```python
from build123d import *

# Parameters (mm, degrees)
SKETCH1_W           = 70
SKETCH1_H           = 154.713144252
SKETCH1_R           = 2.75
SKETCH1_R_2         = 14
BOSS_EXTRUDE1_DEPTH = 5
SKETCH1_4_W         = 70
SKETCH1_4_H         = 154.713144252
SKETCH1_4_R         = 2.75
SKETCH1_4_R_2       = 14
SKETCH1_4_H_2       = 118
SKETCH1_4_R_3       = 5
BOSS_EXTRUDE2_DEPTH = 5
SKETCH2_W           = 70
SKETCH2_H           = 57.356572126
CUT_EXTRUDE1_DEPTH  = 10


with BuildPart() as part:
    # Sketch1 → Boss-Extrude1 (new body)
    with BuildSketch(Plane.XY):
        with Locations((-1.450472168, 0)):
            Rectangle(SKETCH1_W, SKETCH1_H)
        with Locations((-18.5, 57.356572126)):
            Circle(SKETCH1_R, mode=Mode.SUBTRACT)
        with Locations((18.5, 57.356572126)):
            Circle(SKETCH1_R, mode=Mode.SUBTRACT)
        with Locations((-26.450472168, 10)):
            Circle(SKETCH1_R, mode=Mode.SUBTRACT)
        with Locations((26.450472168, 10)):
            Circle(SKETCH1_R, mode=Mode.SUBTRACT)
        with Locations((26.450472168, -10)):
            Circle(SKETCH1_R, mode=Mode.SUBTRACT)
        with Locations((-26.450472168, -10)):
            Circle(SKETCH1_R, mode=Mode.SUBTRACT)
        with Locations((0, 57.356572126)):
            Circle(SKETCH1_R_2, mode=Mode.SUBTRACT)
        with BuildLine():
            Line((-13.95, -33.643427874), (-13.95, -40.643427874))
            ThreePointArc((-13.95, -40.643427874), (-15.5, -42.193427874), (-17.05, -40.643427874))
            Line((-17.05, -40.643427874), (-17.05, -33.643427874))
            ThreePointArc((-17.05, -33.643427874), (-15.5, -32.093427874), (-13.95, -33.643427874))
        make_face(mode=Mode.SUBTRACT)
        with BuildLine():
            Line((17.05, -33.643427874), (17.05, -40.643427874))
            ThreePointArc((17.05, -40.643427874), (15.5, -42.193427874), (13.95, -40.643427874))
            Line((13.95, -40.643427874), (13.95, -33.643427874))
            ThreePointArc((13.95, -33.643427874), (15.5, -32.093427874), (17.05, -33.643427874))
        make_face(mode=Mode.SUBTRACT)
        with BuildLine():
            Line((17.05, -64.643427874), (17.05, -71.643427874))
            ThreePointArc((17.05, -71.643427874), (15.5, -73.193427874), (13.95, -71.643427874))
            Line((13.95, -71.643427874), (13.95, -64.643427874))
            ThreePointArc((13.95, -64.643427874), (15.5, -63.093427874), (17.05, -64.643427874))
        make_face(mode=Mode.SUBTRACT)
        with BuildLine():
            Line((-13.95, -64.643427874), (-13.95, -71.643427874))
            ThreePointArc((-13.95, -71.643427874), (-15.5, -73.193427874), (-17.05, -71.643427874))
            Line((-17.05, -71.643427874), (-17.05, -64.643427874))
            ThreePointArc((-17.05, -64.643427874), (-15.5, -63.093427874), (-13.95, -64.643427874))
        make_face(mode=Mode.SUBTRACT)
        with BuildLine():
            Line((-12, -56.143427874), (-12, -49.143427874))
            ThreePointArc((-12, -49.143427874), (0, -37.143427874), (12, -49.143427874))
            Line((12, -49.143427874), (12, -56.143427874))
            ThreePointArc((12, -56.143427874), (0, -68.143427874), (-12, -56.143427874))
        make_face(mode=Mode.SUBTRACT)
    extrude(amount=BOSS_EXTRUDE1_DEPTH)

    # Sketch1_4 → Boss-Extrude2 (add)
    # profile 1 of 3: a face of its own
    with BuildSketch(Plane.XY):
        with Locations((-1.450472168, 0)):
            Rectangle(SKETCH1_4_W, SKETCH1_4_H)
        with Locations((-26.450472168, -10)):
            Circle(SKETCH1_4_R, mode=Mode.SUBTRACT)
        with BuildLine():
            ThreePointArc((-17.05, -64.643427874), (-15.5, -63.093427874), (-13.95, -64.643427874))
            Line((-13.95, -64.643427874), (-13.95, -71.643427874))
            ThreePointArc((-13.95, -71.643427874), (-15.5, -73.193427874), (-17.05, -71.643427874))
            Line((-17.05, -71.643427874), (-17.05, -64.643427874))
        make_face(mode=Mode.SUBTRACT)
        with BuildLine():
            ThreePointArc((-17.05, -33.643427874), (-15.5, -32.093427874), (-13.95, -33.643427874))
            Line((-13.95, -33.643427874), (-13.95, -40.643427874))
            ThreePointArc((-13.95, -40.643427874), (-15.5, -42.193427874), (-17.05, -40.643427874))
            Line((-17.05, -40.643427874), (-17.05, -33.643427874))
        make_face(mode=Mode.SUBTRACT)
        with Locations((-26.450472168, 10)):
            Circle(SKETCH1_4_R, mode=Mode.SUBTRACT)
        with Locations((-18.5, 57.356572126)):
            Circle(SKETCH1_4_R, mode=Mode.SUBTRACT)
        with BuildLine():
            ThreePointArc((12, -56.143427874), (0, -68.143427874), (-12, -56.143427874))
            Line((-12, -56.143427874), (-12, -49.143427874))
            ThreePointArc((-12, -49.143427874), (0, -37.143427874), (12, -49.143427874))
            Line((12, -49.143427874), (12, -56.143427874))
        make_face(mode=Mode.SUBTRACT)
        with BuildLine():
            ThreePointArc((13.95, -64.643427874), (15.5, -63.093427874), (17.05, -64.643427874))
            Line((17.05, -64.643427874), (17.05, -71.643427874))
            ThreePointArc((17.05, -71.643427874), (15.5, -73.193427874), (13.95, -71.643427874))
            Line((13.95, -71.643427874), (13.95, -64.643427874))
        make_face(mode=Mode.SUBTRACT)
        with BuildLine():
            ThreePointArc((13.95, -33.643427874), (15.5, -32.093427874), (17.05, -33.643427874))
            Line((17.05, -33.643427874), (17.05, -40.643427874))
            ThreePointArc((17.05, -40.643427874), (15.5, -42.193427874), (13.95, -40.643427874))
            Line((13.95, -40.643427874), (13.95, -33.643427874))
        make_face(mode=Mode.SUBTRACT)
        with Locations((26.450472168, -10)):
            Circle(SKETCH1_4_R, mode=Mode.SUBTRACT)
        with Locations((0, 57.356572126)):
            Circle(SKETCH1_4_R_2, mode=Mode.SUBTRACT)
        with Locations((26.450472168, 10)):
            Circle(SKETCH1_4_R, mode=Mode.SUBTRACT)
        with Locations((18.5, 57.356572126)):
            Circle(SKETCH1_4_R, mode=Mode.SUBTRACT)
    # profile 2 of 3: a face of its own
    with BuildSketch(Plane.XY):
        with Locations((-1.450472168, 136.356572126)):
            Rectangle(SKETCH1_4_W, SKETCH1_4_H_2)
        with Locations((-16.991825546, 182.387739686)):
            Circle(SKETCH1_4_R, mode=Mode.SUBTRACT)
        with BuildLine():
            ThreePointArc((-6, 119.856572126), (0, 125.856572126), (6, 119.856572126))
            Line((6, 119.856572126), (6, 94.856572126))
            ThreePointArc((6, 94.856572126), (0, 88.856572126), (-6, 94.856572126))
            Line((-6, 94.856572126), (-6, 119.856572126))
        make_face(mode=Mode.SUBTRACT)
        with Locations((14.09088121, 182.387739686)):
            Circle(SKETCH1_4_R, mode=Mode.SUBTRACT)
    # profile 3 of 3: a face of its own
    with BuildSketch(Plane.XY):
        with Locations((0, 57.356572126)):
            Circle(SKETCH1_4_R_3)
    extrude(amount=BOSS_EXTRUDE2_DEPTH)


with BuildPart() as boss_extrude2_kept_piece:
    # of the separate pieces the step leaves, the one the design keeps (boss_extrude2_pieces_kept)
    add(part.part.solids().sort_by_distance((-36.450472168, -77.356572126, 0))[0])

    # Sketch2 → Cut-Extrude1 (cut)
    with BuildSketch(Plane.XY.offset(5)):
        with Locations((-1.450472168, -48.678286063)):
            Rectangle(SKETCH2_W, SKETCH2_H)
        with BuildLine():
            Line((-13.95, -64.643427874), (-13.95, -71.643427874))
            ThreePointArc((-13.95, -71.643427874), (-15.5, -73.193427874), (-17.05, -71.643427874))
            Line((-17.05, -71.643427874), (-17.05, -64.643427874))
            ThreePointArc((-17.05, -64.643427874), (-15.5, -63.093427874), (-13.95, -64.643427874))
        make_face(mode=Mode.SUBTRACT)
        with BuildLine():
            Line((-13.95, -33.643427874), (-13.95, -40.643427874))
            ThreePointArc((-13.95, -40.643427874), (-15.5, -42.193427874), (-17.05, -40.643427874))
            Line((-17.05, -40.643427874), (-17.05, -33.643427874))
            ThreePointArc((-17.05, -33.643427874), (-15.5, -32.093427874), (-13.95, -33.643427874))
        make_face(mode=Mode.SUBTRACT)
        with BuildLine():
            Line((-12, -56.143427874), (-12, -49.143427874))
            ThreePointArc((-12, -49.143427874), (0, -37.143427874), (12, -49.143427874))
            Line((12, -49.143427874), (12, -56.143427874))
            ThreePointArc((12, -56.143427874), (0, -68.143427874), (-12, -56.143427874))
        make_face(mode=Mode.SUBTRACT)
        with BuildLine():
            Line((17.05, -64.643427874), (17.05, -71.643427874))
            ThreePointArc((17.05, -71.643427874), (15.5, -73.193427874), (13.95, -71.643427874))
            Line((13.95, -71.643427874), (13.95, -64.643427874))
            ThreePointArc((13.95, -64.643427874), (15.5, -63.093427874), (17.05, -64.643427874))
        make_face(mode=Mode.SUBTRACT)
        with BuildLine():
            Line((17.05, -33.643427874), (17.05, -40.643427874))
            ThreePointArc((17.05, -40.643427874), (15.5, -42.193427874), (13.95, -40.643427874))
            Line((13.95, -40.643427874), (13.95, -33.643427874))
            ThreePointArc((13.95, -33.643427874), (15.5, -32.093427874), (17.05, -33.643427874))
        make_face(mode=Mode.SUBTRACT)
    extrude(amount=-CUT_EXTRUDE1_DEPTH, mode=Mode.SUBTRACT)


solid = boss_extrude2_kept_piece.part
```
Input: part model. Units: mm. Frame: model coordinates. A direction names the side the tool comes from. Coordinates: 2 decimals unless noted, no trailing zeros. Loops run counter-clockwise (first coordinate to the right, second up) from the corner with the lowest first, then second, coordinate; pieces in that order, holes last. Notation, with made-up numbers: M 10,31.5 L 40,31.5 A4 ccw 40,36.5 Z; hole C 87,30 d10. An arc over 180 degrees is marked long. Use a Markdown table: item, result. Add a question column.
1) Section B-B, the plane x = 0. Return the cut outline in (y, z).
2) Section C-C, the plane x = -11. Return the cut outline in (y, z).
3) Section A-A, the plane y = 10. Return the cut outline in (x, z), plus the area to 3 significant figures.
4) Line query: L1, parallel to Y at x = -26.5, z = 4.4; L2, parallel to X at y = 8, z = 3.4; L3, parallel to Y at x = -18.5, z = 2.3. Output: solid intervals per line, ascending. Write a range as from..to.
5) Section D-D, the plane z = 3.6. Give the number of separate pieces and of enclosed holes in the cut face, plus the area to 3 significant figures.
6) Draft query along Y for faces 3 (the flat face through (-2, 195.357, 2)), 4 (the cylindrical face through (-20.68, 55.68, 2.46)), 5 (the flat face through (33.55, 86, 2)), 6 (the flat face through (6, 108, 2)). Return one class per face: +Y half, -Y half, draft (parallel to the pull), parting line (faces both ways), or undercut.
7) Set-up query: faces 1 (the cylindrical face through (0.132, 88.858, 2.465)), 2 (the flat face through (-10, 89, 5)). Return all of +Z, -Z, +X, -X, +Y, -Y with unobstructed straight access to the full face (end or side cutting, diameter ignored); none if empty.
Answer below:
| question | item | result |
|---|---|---|
| 1 | outline | M -20,0 L 43.36,0 L 43.36,5 L -20,5 Z; M 71.36,0 L 88.86,0 L 88.86,5 L 71.36,5 Z; M 125.86,0 L 195.36,0 L 195.36,5 L 125.86,5 Z |
| 2 | outline | M -20,0 L 48.7,0 L 48.7,5 L -20,5 Z; M 66.02,0 L 195.36,0 L 195.36,5 L 66.02,5 Z |
| 3 | outline | M -36.45,0 L -29.2,0 L -29.2,5 L -36.45,5 Z; M -23.7,0 L 23.7,0 L 23.7,5 L -23.7,5 Z; M 29.2,0 L 33.55,0 L 33.55,5 L 29.2,5 Z |
| 3 | area | 295 mm2 |
| 4 | L1 | -20..-12.75, -7.25..7.25, 12.75..195.36 |
| 4 | L2 | -36.45..-28.34, -24.56..24.56, 28.34..33.55 |
| 4 | L3 | -20..54.61, 60.11..180.09, 184.69..195.36 |
| 5 | separate pieces | 1 |
| 5 | enclosed holes | 10 |
| 5 | area | 13,900 mm2 |
| 6 | face 3 | +Y half |
| 6 | face 4 | undercut |
| 6 | face 5 | draft |
| 6 | face 6 | undercut |
| 7 | face 1 | +Z, -Z |
| 7 | face 2 | +Z, +X, -X, +Y, -Y |
